Read the model definition and answer for the solid it produces. Units are mm, in the model's axes. A direction names the side the tool comes from. Coordinates: 2 decimals unless noted, no trailing zeros. Write each loop counter-clockwise with the first axis right and the second up, starting at its lowest first coordinate (ties: lowest second). Pieces come first, ordered by that corner, then holes. Notation, with made-up numbers: (30.25, 47.25) -> (47.25, 47.25) arc R23 ccw to (47.25, 84.25) -> close; hole circle Ø4 at (81.5, 58). An arc over 180 degrees is marked (long way). Answer as a JSON object with one key per item and string values. Group by question number.
(1) Flat-ended cylindrical pins translate along their axes: P1, Ø1.5, axis at y = 2, z = -2, coming from the -X side; P2, Ø1, axis at x = 3, y = 1.5, coming from the +Z side; P3, Ø1.5, axis at y = -1, z = -5, coming from the -X side; P4, Ø1, axis at x = 4.5, z = -4, coming from the -Y side. Find the tip coordinate at first contact, or state that the pin passes through.
(2) Find section D-D (y = 1.6). Give the vertices of the cut face in (x, z), then the cut area to 3 significant figures.
(3) Straight lines are drawn through the part: L1, parallel to Y at x = 7, z = -2.5; L2, parallel to Y at x = 4, z = -4; L3, parallel to X at y = 0.2, z = -3.75. For each, find the intervals that lie inside material, in ascending order.
(4) Find section C-C (x = 4). Give the vertices of the cut face in (y, z).
(5) Find section B-B (z = -4.75). Give the vertices of the cut face in (x, y).
(6) Find section A-A (y = 0.25). Give the vertices of the cut face in (x, z), then the cut area to 3 significant figures.
(7) Which of the six approach directions +Z, -Z, +X, -X, +Y, -Y give full straight-line access (tool end or side, diameter ignored) to faces 4 (the face through (5, 3, -4)), 5 (the face through (2.94, 0.2, -2.36)), 6 (the face through (3, 0, -2)), 7 (the face through (5.08, 2.8, -5.29)), 8 (the face through (4, -1, -8))?
(8) For a pull along X with two mould halves and no side action, classify faces 1 (the face through (1.49, -1.48, -7.49)), 2 (the face through (7.7, 1.5, -4.1)), 3 (the face through (5.081, 2.803, -3.293)) as +X half, -X half, draft (parallel to the pull), parting line (faces both ways), or undercut.
from build123d import *

# Parameters (mm, degrees)
SKETCH1_W               = 8
SKETCH1_H               = 8
BOSS_EXTRUDE1_DEPTH     = 3
CUT_EXTRUDE1_DEPTH      = 12.704699911
CUT_EXTRUDE1_DEPTH_BACK = 12.704699911
CUT_EXTRUDE2_DEPTH      = 11
SKETCH4_R               = 1.75
CUT_EXTRUDE3_DEPTH      = 0.4
SKETCH5_W               = 8
SKETCH5_H               = 1
BOSS_EXTRUDE2_DEPTH     = 2
FILLET1_R               = 4
CUT_EXTRUDE4_DEPTH      = 0.4


with BuildPart() as part:
    # Sketch1 → Boss-Extrude1 (new body)
    with BuildSketch(Plane(origin=(0, 0, 0), x_dir=(1, 0, 0), z_dir=(0, 1, 0))):
        with Locations((4, 4)):
            Rectangle(SKETCH1_W, SKETCH1_H)
    extrude(amount=BOSS_EXTRUDE1_DEPTH)

    # Sketch2 → Cut-Extrude1 (cut, two sides: drawn at the far end of the back side and taken through both)
    with BuildSketch(Plane.XY.offset(-CUT_EXTRUDE1_DEPTH_BACK)):
        Polygon((0, 0), (0.6, 3), (0, 3), align=None)
        Polygon((8, 0), (7.4, 3), (8, 3), align=None)
    extrude(amount=CUT_EXTRUDE1_DEPTH + CUT_EXTRUDE1_DEPTH_BACK, mode=Mode.SUBTRACT)

    # Sketch3 → Cut-Extrude2 (cut)
    with BuildSketch(Plane(origin=(0, 0, 0), x_dir=(0, 0, -1), z_dir=(1, 0, 0))):
        Polygon((0, 0), (0.6, 3), (0, 3), align=None)
        Polygon((8, 3), (7.4, 3), (8, 0), align=None)
    extrude(amount=CUT_EXTRUDE2_DEPTH, mode=Mode.SUBTRACT)

    # Sketch4 → Cut-Extrude3 (cut)
    with BuildSketch(Plane.XZ):
        with Locations(Location((4, -3.75, 0), (0, 0, 270))):
            Circle(SKETCH4_R)
    extrude(amount=-CUT_EXTRUDE3_DEPTH, mode=Mode.SUBTRACT)

    # Sketch5 → Boss-Extrude2 (add)
    with BuildSketch(Plane.XZ):
        with Locations((4, -7.5)):
            Rectangle(SKETCH5_W, SKETCH5_H)
    extrude(amount=BOSS_EXTRUDE2_DEPTH)

    # Fillet1
    # the kernel refuses this fillet: 4 mm, written as the material it takes off along each edge
    with BuildSketch(Plane(origin=(8, -2, -16.660254038), x_dir=(0, 1, 0), z_dir=(0, 0, 1)), Plane(origin=(0, -2, 1.660254038), x_dir=(0, 1, 0), z_dir=(0, 0, -1))) as fillet1_piece_1:
        with BuildLine():
            CenterArc((4, 3.464101615), FILLET1_R, 180, 60)
            Line((0, 3.464101615), (-0.08, 3.464101615))
            Line((-0.08, 3.464101615), (-0.08, 0))
            Line((-0.08, 0), (0, -0.08))
            ThreePointArc((0, -0.08), (1, -0.08), (1.96, -0.069282032))
            Line((1.96, -0.069282032), (2, 0))
        make_face()
    extrude(amount=18.320508076, mode=Mode.SUBTRACT)

    # Sketch6 → Cut-Extrude4 (cut)
    with BuildSketch(Plane(origin=(0, 3, 0), x_dir=(1, 0, 0), z_dir=(0, 1, 0))):
        Polygon((2.312898911, 2.049121591), (2.312898911, 6.049121591), (3.08212968, 6.049121591), (3.08212968, 4.258256206), (4.768828398, 6.049121591), (5.825719424, 6.049121591), (4.306488654, 4.502647232), (5.877001475, 2.049121591), (4.852161731, 2.049121591), (3.723155321, 3.907294667), (3.08212968, 3.255051078), (3.08212968, 2.049121591), align=None)
    extrude(amount=-CUT_EXTRUDE4_DEPTH, mode=Mode.SUBTRACT)


solid = part.part
Results below:
{
 "1": {"P1": "stops at x = 0.25", "P2": "stops at z = -0.2", "P3": "passes through", "P4": "stops at y = 0.4"},
 "2": {"outline": "(0.32, -7.68) -> (7.68, -7.68) -> (7.68, -0.32) -> (0.32, -0.32) -> close", "area": "54.2 mm2"},
 "3": {"L1": "y = 0 to 3", "L2": "y = 0.4 to 2.6", "L3": "x = 0.04 to 2.25, 5.75 to 7.96"},
 "4": {"outline": "(-2, -8) -> (0, -8) -> (3, -7.4) -> (3, -5.23) -> (2.6, -5.23) -> (2.6, -3.45) -> (3, -3.45) -> (3, -0.6) -> (0, 0) -> (0, -2) -> (0.4, -2) -> (0.4, -5.5) -> (0, -5.5) -> (0, -7) -> (-2, -7) -> close"},
 "5": {"outline": "(0, 0) -> (2.56, 0) -> (2.56, 0.4) -> (5.44, 0.4) -> (5.44, 0) -> (8, 0) -> (7.4, 3) -> (4.55, 3) -> (4.55, 2.6) -> (3.55, 2.6) -> (3.55, 3) -> (3.08, 3) -> (3.08, 2.6) -> (2.31, 2.6) -> (2.31, 3) -> (0.6, 3) -> close"},
 "6": {"outline": "(0.05, -7.95) -> (7.95, -7.95) -> (7.95, -0.05) -> (0.05, -0.05) -> close; hole circle Ø3.5 at (4, -3.75)", "area": "52.8 mm2"},
 "7": {"face 4": "+Z, -Z, +X, -X, +Y", "face 5": "-Y", "face 6": "+Z, +X, -X, -Y", "face 7": "+Y", "face 8": "-Z, +X, -X, +Y, -Y"},
 "8": {"face 1": "-X half", "face 2": "+X half", "face 3": "undercut"}
}
